Source: CAD feature listing. Evaluate the final solid. Frame: model axes, mm. Round coordinates to 2 decimals unless told otherwise and drop trailing zeros. Loops run counter-clockwise (first coordinate to the right, second up) from the corner with the lowest first, then second, coordinate; pieces in that order, holes last. Notation, with made-up numbers: (-1.75, 67.25) - (9.25, 67.25) arc R5 cw to (9.25, 73.25) - close; hole circle Ø6 at (35, 9.5). An arc over 180 degrees is marked (long way). One line per question, with ' | ' between items.
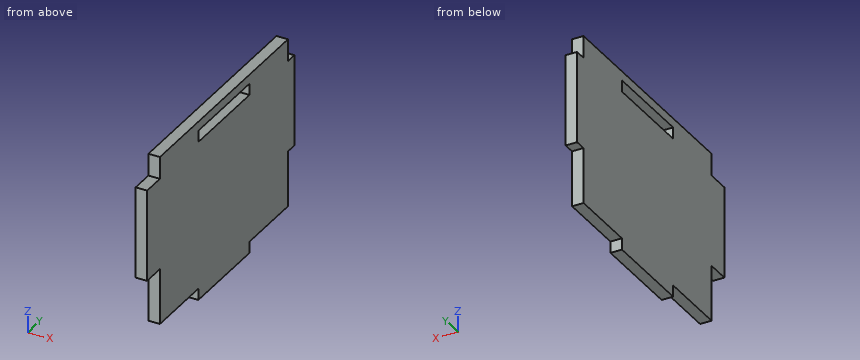
from build123d import *

# Parameters (mm, degrees)
SKETCH1_W           = 2.5
SKETCH1_H           = 20
BOSS_EXTRUDE2_DEPTH = 1.25


with BuildPart() as part:
    # Sketch1 (on Right Plane) → Boss-Extrude2 (new, symmetric)
    with BuildSketch(Plane(origin=(0, 0, 0), x_dir=(0, 0, -1), z_dir=(1, 0, 0))):
        Polygon((4.833333333, 5), (0, 5), (0, 55), (4.833333333, 55), (4.833333333, 57.5), (24.833333333, 57.5), (24.833333333, 55), (37, 55), (37, 40), (39.5, 40), (39.5, 20), (37, 20), (37, 5), (24.833333333, 5), (24.833333333, 0), (4.833333333, 0), align=None)
        with Locations((3.25, 30)):
            Rectangle(SKETCH1_W, SKETCH1_H, mode=Mode.SUBTRACT)
    extrude(amount=BOSS_EXTRUDE2_DEPTH, both=True)


solid = part.part
1. Contact query for flat-ended pins moving along their axis: P1, Ø0.8, axis at x = 0.5, y = 56, coming from the -Z side; P2, Ø0.8, axis at x = 0, z = -37.5, coming from the +Y side; P3, Ø1.2, axis at x = 0.5, z = -2.5, coming from the +Y side. Output: stop coordinate, or through.
Worked out:
P1: stops at z = -24.83 | P2: stops at y = 40 | P3: stops at y = 55
2. Section query C-C, the plane z = -27. Return loops of the section in (x, y).
Worked out:
outline: (-1.25, 5) - (1.25, 5) - (1.25, 55) - (-1.25, 55) - close
3. Section query B-B, the plane x = 0.2. Return loops of the section in (y, z), plus the area to 3 significant figures.
Worked out:
outline: (0, -24.83) - (5, -24.83) - (5, -37) - (20, -37) - (20, -39.5) - (40, -39.5) - (40, -37) - (55, -37) - (55, -24.83) - (57.5, -24.83) - (57.5, -4.83) - (55, -4.83) - (55, 0) - (5, 0) - (5, -4.83) - (0, -4.83) - close; hole (20, -4.5) - (40, -4.5) - (40, -2) - (20, -2) - close | area: 2,000 mm2
4. Section query D-D, the plane y = 50. Return loops of the section in (x, z), plus the area to 3 significant figures.
Worked out:
outline: (-1.25, -37) - (1.25, -37) - (1.25, 0) - (-1.25, 0) - close | area: 92.5 mm2
5. Section query A-A, the plane y = 28.5. Return loops of the section in (x, z), plus the area to 3 significant figures.
Worked out:
outline: (-1.25, -39.5) - (1.25, -39.5) - (1.25, -4.5) - (-1.25, -4.5) - close; (-1.25, -2) - (1.25, -2) - (1.25, 0) - (-1.25, 0) - close | area: 92.5 mm2
6. Material intervals for probe 1 along Z at (x, y) = (-0.3, 21.5); probe 2 along Z at (x, y) = (0.75, 45); probe 3 along Y at (x, z) = (1.15, -29), sorted ascending.
Worked out:
probe 1: z = -39.5 to -4.5, -2 to 0 | probe 2: z = -37 to 0 | probe 3: y = 5 to 55
